CAD build for the part. Positions are in the model's coordinates, mm. Face numbers are marked on the shaded views. Coordinates: 2 decimals unless noted, no trailing zeros. Write each loop counter-clockwise with the first axis right and the second up, starting at its lowest first coordinate (ties: lowest second). Pieces come first, ordered by that corner, then holes. Notation, with made-up numbers: M -20,-15.5 L 35,-15.5 A18 ccw 35,5.5 Z; hole C -21,33 d8. An arc over 180 degrees is marked long. Put each result on its own line as item: value. Start each with the question number.
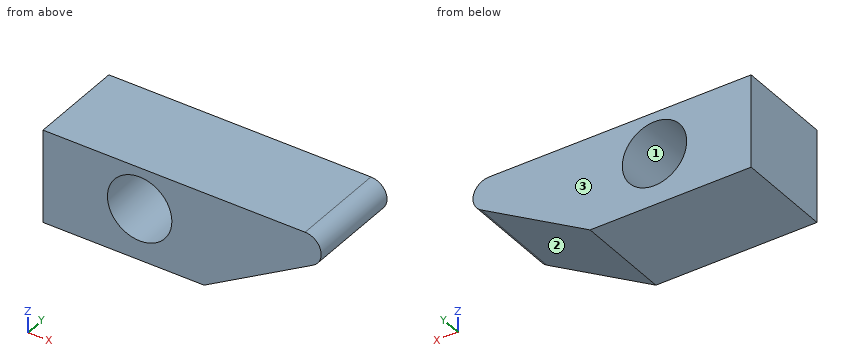
```python
from build123d import *

# Parameters (mm, degrees)
F1_DEPTH = 30
F2_R     = 10
F3_DEPTH = 30
F4_R     = 5


with BuildPart() as f1:
    # F0 (on Front) → F1 (new body)
    with BuildSketch(Plane.XZ):
        Polygon((0, 28.867513), (0, 0), (50, 0), (100, 28.867513), align=None)
    extrude(amount=F1_DEPTH)

    # F2 (on face) → F3 (cut, through all)
    with BuildSketch(Plane.XZ.offset(30)):
        with Locations((30, 16)):
            Circle(F2_R)
    extrude(amount=-F3_DEPTH, mode=Mode.SUBTRACT)

    # F4
    f4_edges = [f1.edges().sort_by_distance(p)[0] for p in [
        (100, -15, 28.867513),
    ]]
    fillet(f4_edges, radius=F4_R)


solid = f1.part
```
(1) Slice it at C-C, the plane y = -28. Write the cut outline in (x, z), then the cut area to 3 significant figures.
(2) Two-plate mould, pull along Z, no slides. Class the marked faces 1, 2 and 3: +Z half, -Z half, draft (parallel to the pull), parting line (faces both ways), or undercut.
(3) Slice it at D-D, the plane x = 79. Write the cut outline in (y, z), then the cut area to 3 significant figures.
(4) Drill centre lines: line 1 (Z direction, x = 30, y = -23.5); line 2 (X direction, y = -19.5, z = 11.75); line 3 (X direction, y = -18.75, z = 7). Where is each one in solid material? Low to high. Write a range as [from, to].
(5) Slice it at A-A, the plane x = 30. Write the cut outline in (y, z).
(6) Drop flat-ended pins along their axis: pin 1 (3 mm diameter, centred on y = -14.5, z = 10, fed in from +X); pin 2 (2 mm diameter, centred on y = -19, z = 14.5, fed in from +X); pin 3 (6 mm diameter, centred on x = 73, z = 11.5, fed in from -Y); pin 4 (5 mm diameter, centred on x = 55, y = -22.5, fed in from -Z). Give the stop position or say it passes through.
(7) Slice it at B-B, the plane z = 10. Write the cut outline in (x, y), then the cut area to 3 significant figures.
Result set:
1. outline: M 0,0 L 50,0 L 83.84,19.54 A5 ccw 81.34,28.87 L 0,28.87 Z; hole C 30,16 d20
1. area: 1,790 mm^2
2. face 1: undercut
2. face 2: -Z half
2. face 3: draft
3. outline: M -30,16.74 L 0,16.74 L 0,28.87 L -30,28.87 Z
3. area: 364 mm^2
4. line 1: z = [0, 6], [26, 28.87]
4. line 2: x = [0, 20.95], [39.05, 70.35]
4. line 3: x = [0, 25.64], [34.36, 62.12]
5. outline: M -30,0 L 0,0 L 0,6 L -30,6 Z; M -30,26 L 0,26 L 0,28.87 L -30,28.87 Z
6. pin 1: stops at x = 69.92
6. pin 2: stops at x = 76.85
6. pin 3: stops at y = -30
6. pin 4: stops at z = 1.44
7. outline: M 0,-30 L 22,-30 L 22,0 L 0,0 Z; M 38,-30 L 67.32,-30 L 67.32,0 L 38,0 Z
7. area: 1,540 mm^2
